Design review of the part built by this model. Coordinates are the model's own, in mm. A direction names the side the tool comes from. Give positions to 0.01 mm unless a question says otherwise; leave off trailing zeros. Write each loop counter-clockwise with the first axis right and the second up, starting at its lowest first coordinate (ties: lowest second). Pieces come first, ordered by that corner, then holes. Notation, with made-up numbers: M 45.5,21 L 100.5,21 A24 cw 100.5,43 Z; hole C 49.25,80 d3. An arc over 180 degrees is marked long. Answer in a Markdown table with one row per item.
```python
from build123d import *

# Parameters (mm, degrees)
SKETCH2_W               = 279.4
SKETCH2_H               = 279.4
BOSS_EXTRUDE1_DEPTH     = 9.525
SKETCH4_W               = 9.525
SKETCH4_H               = 25.4
BOSS_EXTRUDE3_DEPTH     = 9.525
LPATTERN2_COUNT         = 5
LPATTERN2_PITCH         = 50.8
MIRROR2_COPY_1_SKETCH_W = 9.525
MIRROR2_COPY_1_SKETCH_H = 25.4
MIRROR2_COPY_1_DEPTH    = 9.525
MIRROR2_COPY_2_SKETCH_W = 9.525
MIRROR2_COPY_2_SKETCH_H = 25.4
MIRROR2_COPY_2_DEPTH    = 9.525
MIRROR2_COPY_3_SKETCH_W = 9.525
MIRROR2_COPY_3_SKETCH_H = 25.4
MIRROR2_COPY_3_DEPTH    = 9.525
MIRROR2_COPY_4_SKETCH_W = 9.525
MIRROR2_COPY_4_SKETCH_H = 25.4
MIRROR2_COPY_4_DEPTH    = 9.525
SKETCH5_W               = 25.4
SKETCH5_H               = 9.525
BOSS_EXTRUDE4_DEPTH     = 9.525
LPATTERN3_COUNT         = 5
LPATTERN3_PITCH         = 50.8
SKETCH6_R               = 2.3368
CUT_EXTRUDE1_DEPTH      = 10.525


with BuildPart() as part:
    # Sketch2 → Boss-Extrude1 (new body)
    with BuildSketch(Plane.XY):
        Rectangle(SKETCH2_W, SKETCH2_H)
    extrude(amount=BOSS_EXTRUDE1_DEPTH)

    # Sketch4 → Boss-Extrude3 (add)
    with BuildSketch(Plane(origin=(139.7, 0, 0), x_dir=(0, 0, -1), z_dir=(1, 0, 0))):
        with Locations((-4.7625, -101.6)):
            Rectangle(SKETCH4_W, SKETCH4_H)
    boss_extrude3 = extrude(amount=BOSS_EXTRUDE3_DEPTH)

    # LPattern2: Boss-Extrude3 ×5
    with Locations(*[(0, i * LPATTERN2_PITCH, 0) for i in range(1, LPATTERN2_COUNT)]):
        add(boss_extrude3)

    # Mirror2: Boss-Extrude3 across plane
    add(boss_extrude3.mirror(Plane(origin=(0, 0, 0), x_dir=(0, 0, 1), z_dir=(1, 0, 0))))

    # Mirror2 copy 1 sketch → Mirror2 copy 1 (add)
    with BuildSketch(Plane(origin=(-139.7, 50.8, 0), x_dir=(0, 0, -1), z_dir=(-1, 0, 0))):
        with Locations((-4.7625, 101.6)):
            Rectangle(MIRROR2_COPY_1_SKETCH_W, MIRROR2_COPY_1_SKETCH_H)
    extrude(amount=MIRROR2_COPY_1_DEPTH)

    # Mirror2 copy 2 sketch → Mirror2 copy 2 (add)
    with BuildSketch(Plane(origin=(-139.7, 101.6, 0), x_dir=(0, 0, -1), z_dir=(-1, 0, 0))):
        with Locations((-4.7625, 101.6)):
            Rectangle(MIRROR2_COPY_2_SKETCH_W, MIRROR2_COPY_2_SKETCH_H)
    extrude(amount=MIRROR2_COPY_2_DEPTH)

    # Mirror2 copy 3 sketch → Mirror2 copy 3 (add)
    with BuildSketch(Plane(origin=(-139.7, 152.4, 0), x_dir=(0, 0, -1), z_dir=(-1, 0, 0))):
        with Locations((-4.7625, 101.6)):
            Rectangle(MIRROR2_COPY_3_SKETCH_W, MIRROR2_COPY_3_SKETCH_H)
    extrude(amount=MIRROR2_COPY_3_DEPTH)

    # Mirror2 copy 4 sketch → Mirror2 copy 4 (add)
    with BuildSketch(Plane(origin=(-139.7, 203.2, 0), x_dir=(0, 0, -1), z_dir=(-1, 0, 0))):
        with Locations((-4.7625, 101.6)):
            Rectangle(MIRROR2_COPY_4_SKETCH_W, MIRROR2_COPY_4_SKETCH_H)
    extrude(amount=MIRROR2_COPY_4_DEPTH)

    # Sketch5 → Boss-Extrude4 (add)
    with BuildSketch(Plane.XZ.offset(139.7)):
        with Locations((-101.6, 4.7625)):
            Rectangle(SKETCH5_W, SKETCH5_H)
    boss_extrude4 = extrude(amount=BOSS_EXTRUDE4_DEPTH)

    # LPattern3: Boss-Extrude4 ×5
    with Locations(*[(i * LPATTERN3_PITCH, 0, 0) for i in range(1, LPATTERN3_COUNT)]):
        add(boss_extrude4)

    # Sketch6 → Cut-Extrude1 (cut, through all)
    with BuildSketch(Plane.XY.offset(9.525)):
        with Locations((114.3, 129.3876)):
            Circle(SKETCH6_R)
        with Locations((77.7748, 129.3876)):
            Circle(SKETCH6_R)
        with Locations((96.0374, 129.3876)):
            Circle(SKETCH6_R)
    cut_extrude1 = extrude(amount=-CUT_EXTRUDE1_DEPTH, mode=Mode.SUBTRACT)

    # Mirror3: Cut-Extrude1 across plane
    add(cut_extrude1.mirror(Plane(origin=(0, 0, 0), x_dir=(0, 0, 1), z_dir=(1, 0, 0))), mode=Mode.SUBTRACT)


solid = part.part
```
1) Insertion check: P1, Ø3, axis at x = 143.5, z = 3.5, coming from the -Y side; P2, Ø5, axis at x = -143.5, z = 4, coming from the +Y side; P3, Ø3, axis at x = -133, z = 4, coming from the -Y side; P4, Ø4, axis at x = 77.77, y = 129.39, coming from the -Z side. Each pin has a flat end and moves straight along its axis. Give the tip position at first contact, or say it passes through.
Geometry says:
| item | result |
|---|---|
| P1 | y = -114.3 |
| P2 | y = 114.3 |
| P3 | y = -139.7 |
| P4 | through |
2) Add section A-A (z = 3.75). Count the separate pieces of the cut face and the enclosed holes in it, and give its area (3 significant figures).
Geometry says:
| item | result |
|---|---|
| separate pieces | 1 |
| enclosed holes | 6 |
| area | 81,600 mm^2 |
3) The part is to be moulded in two halves that separate along Y. For faces 1 (the face through (-2, 139.7, 5)), 2 (the face through (114.3, -144, 5)), 3 (the face through (-144, 63.5, 5)), 4 (the face through (101, -149.225, 5)), say which applies: released by +Y, released by -Y, zero draft, split by the parting line, or undercut.
Geometry says:
| item | result |
|---|---|
| face 1 | released by +Y |
| face 2 | zero draft |
| face 3 | undercut |
| face 4 | released by -Y |
4) For faces 5 (the face through (76, -139.7, 5)), 6 (the face through (-144, -88.9, 5)), 7 (the face through (-127, -139.7, 5)), 8 (the face through (-139.7, 127, 5)), 9 (the face through (144, -88.9, 5)), list the 3-axis set-ups (+Z, -Z, +X, -X, +Y, -Y) from which the entire face can be reached by the end or side of a thin tool; tool diameter is ignored.
Geometry says:
| item | result |
|---|---|
| face 5 | +Z, -Z, -Y |
| face 6 | +Z, -Z, -X |
| face 7 | +Z, -Z, -X, -Y |
| face 8 | +Z, -Z, -X, +Y |
| face 9 | +Z, -Z, +X |
5) Add section B-B (y = -33). Write out the cut boundary in (x, z) (3 decimals), and give its area (3 significant figures).
Geometry says:
| item | result |
|---|---|
| outline | M -139.7,0 L 139.7,0 L 139.7,9.525 L -139.7,9.525 Z |
| area | 2,660 mm^2 |
6) To check wall thickness, follow probe 1 along Y at (x, z) = (119, 5.25); probe 2 along Y at (x, z) = (-113.5, 4.5) (3 decimals). State the ranges of each line that lie inside material, in increasing order. Write a range as [from, to].
Geometry says:
| item | result |
|---|---|
| probe 1 | [-139.7, 139.7] |
| probe 2 | [-149.225, 127.192], [131.583, 139.7] |
